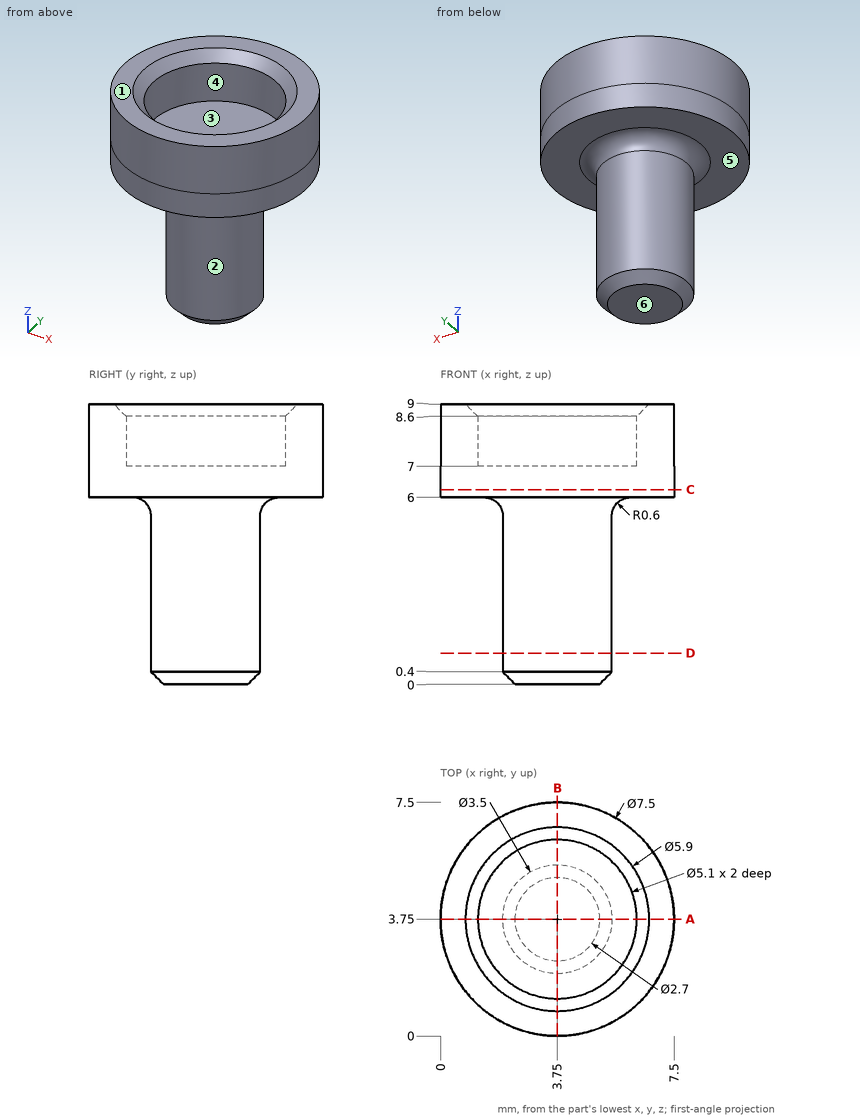
Part print with two shaded views. Sizes in mm from the minimum x, y, z corner. A direction names the side the tool comes from. Round coordinates to 2 decimals unless told otherwise and drop trailing zeros. Order: outer loops, then holes, each group sorted by start corner. A loop starts at its lowest first (then second) coordinate and runs counter-clockwise, first axis right, second up. Notation, with made-up numbers: (46.25, 75) - (94.25, 75) arc R19 cw to (94.25, 79) - close; hole circle Ø7 at (49.25, -28.5). An arc over 180 degrees is marked (long way). Return JSON: item names as keys, results as strings.
(1) Pull direction X, two halves, no side cores. Call the marked faces 1, 2 and 3: +X half, -X half, draft (parallel to the pull), parting line (faces both ways), or undercut.
Answer key:
{"face 1": "draft", "face 2": "parting line", "face 3": "undercut"}
(2) Cut at C-C (z = 6.25). Give the cut face in (x, y), then the cut area to 3 significant figures.
Answer key:
{"outline": "circle Ø7.5 at (3.75, 3.75)", "area": "44.2 mm^2"}
(3) Tool access for the marked faces 4, 5 and 6: list every direction of +Z, -Z, +X, -X, +Y, -Y with a clear straight run to the whole face (end or side of a thin tool).
Answer key:
{"face 4": "+Z", "face 5": "-Z", "face 6": "-Z, +X, -X, +Y, -Y"}
(4) Cut at A-A (y = 3.75). Give the cut face in (x, z), then the cut area to 3 significant figures.
Answer key:
{"outline": "(0, 6) - (1.4, 6) arc R0.6 cw to (2, 5.4) - (2, 0.4) - (2.4, 0) - (5.1, 0) - (5.5, 0.4) - (5.5, 5.4) arc R0.6 cw to (6.1, 6) - (7.5, 6) - (7.5, 9) - (6.7, 9) - (6.3, 8.6) - (6.3, 7) - (1.2, 7) - (1.2, 8.6) - (0.8, 9) - (0, 9) - close", "area": "33.1 mm^2"}
(5) Pin check, flat tips, straight feed: pin 1 Ø4 at (y, z) = (5.5, 3) entering from -X; pin 2 Ø1 at (y, z) = (3, 7) entering from +X; pin 3 Ø2 at (x, z) = (4.5, 4) entering from -Y; pin 4 Ø2 at (x, y) = (4, 4.5) entering from -Z. Stop position of each tip, or through.
Answer key:
{"pin 1": "stops at x = 2", "pin 2": "stops at x = 7.49", "pin 3": "stops at y = 2", "pin 4": "stops at z = 0"}
(6) Cut at D-D (z = 1). Give the cut face in (x, y), then the cut area to 3 significant figures.
Answer key:
{"outline": "circle Ø3.5 at (3.75, 3.75)", "area": "9.62 mm^2"}
(7) Wall check: probe 1 along Y at (x, z) = (3.75, 8.1); probe 2 along Z at (x, y) = (6.5, 2.5); probe 3 along Z at (x, y) = (3.75, 3). Give the ranges that are in metal, low to high. Write a range as from..to.
Answer key:
{"probe 1": "y = 0..1.2, 6.3..7.5", "probe 2": "z = 6..9", "probe 3": "z = 0..7"}
